Part model, mm, in its own coordinate system. A direction names the side the tool comes from. Round coordinates to 2 decimals unless told otherwise and drop trailing zeros. Order: outer loops, then holes, each group sorted by start corner. A loop starts at its lowest first (then second) coordinate and runs counter-clockwise, first axis right, second up. Notation, with made-up numbers: (88.5, 69) - (124.5, 69) arc R29 ccw to (124.5, 97) - close; hole circle Ø3 at (75.5, 25). An arc over 180 degrees is marked (long way). Return JSON: item names as keys, results as strings. Group by question number.
Item 1: Drop flat-ended pins along their axis: pin 1 (2.5 mm diameter, centred on x = 0, y = 14, fed in from +Z); pin 2 (10 mm diameter, centred on y = -10, z = -13.5, fed in from +X); pin 3 (2 mm diameter, centred on x = -11, z = 2.5, fed in from -Y); pin 4 (4 mm diameter, centred on x = -4, z = -44, fed in from -Y). Give the stop position or say it passes through.
Item 2: Saw through at A-A on x = 0. List the corners of the cut face in (y, z).
Item 3: Probe probe 1 along Z at (x, y) = (-9.5, -1.5); probe 2 along Y at (x, z) = (-16, -24.5); probe 3 along X at (y, z) = (15, -8.5) (3 decimals). List the from-to ranges inside material, lowest first.
Item 4: Saw through at B-B on z = -16. List the corners of the cut face in (x, y).
Item 5: Two-plate mould, pull along Y, no slides. Class faces 4 (the face through (-0.29, -2.23, 13.11)), 5 (the face through (-13.23, -5.986, -1.972)), 6 (the face through (0, -8, -47.5)), 7 (the face through (0, 1.5, 15)): released by +Y, released by -Y, zero draft, split by the parting line, or undercut.
Item 6: Tool access for faces 1 (the face through (-6.963, -2.193, -49.817)), 2 (the face through (0, 0, 23)), 3 (the face through (8, 0, 0)): list every direction of +Z, -Z, +X, -X, +Y, -Y with a clear straight run to the whole face (end or side of a thin tool).
Item 7: Saw through at C-C on z = 18.5. List the corners of the cut face in (x, y).
Autodesk Inventor part; units mm, degrees
ref_plane "YZ Plane" through (0, 0, 0) normal (1, 0, 0) x (0, 1, 0)
ref_plane "XZ Plane" through (0, 0, 0) normal (0, 1, 0) x (-1, 0, 0)
ref_plane "XY Plane" through (0, 0, 0) normal (0, 0, 1) x (1, 0, 0)
sketch "Esquisse1" plane through (0, 0, 0) normal (0, 0, 1) x (1, 0, 0)
  circle A0 centre (0, 0) radius 19.2
  dimension "d0" = 38.4
extrude "Extrusion1" add sketch "Esquisse1" against normal blind 47.5
sketch "Esquisse2" plane through (0, 0, 0) normal (0, 0, 1) x (1, 0, 0)
  circle A0 centre (0, 0) radius 19.2
  circle A1 centre (0, 0) radius 7.5
  dimension "d3" = 15
extrude "Extrusion2" add sketch "Esquisse2" along normal blind 3.5 contours A1
sketch "Esquisse3" plane through (0, 0, 3.5) normal (0, 0, 1) x (1, 0, 0)
  circle A0 centre (0, 0) radius 7.5
  circle A1 centre (0, 0) radius 2.25
  dimension "d6" = 4.5
extrude "Extrusion3" add sketch "Esquisse3" along normal blind 19.5 contours A1
sketch "Esquisse4" plane through (0, 0, -47.5) normal (0, 0, -1) x (-1, 0, 0)
  circle A0 centre (0, 0) radius 19.2
  circle A1 centre (0, 0) radius 7.3
  dimension "d9" = 14.6
extrude "Extrusion4" add sketch "Esquisse4" along normal blind 5.7 contours A1
fillet "Congé1" radius 1 1 edges at (7.3, 0, -53.2)
fillet "Congé2" radius 1 1 edges at (-19.2, 0, 0)
sketch "Esquisse6" plane through (0, 0, 23) normal (0, 0, 1) x (1, 0, 0)
  circle A0 centre (0, 0) radius 2.25
  line L0 (-3, 3.5) -> (3, 3.5)
  line L1 (3, 3.5) -> (3, 1.5)
  line L2 (3, 1.5) -> (-3, 1.5)
  line L3 (-3, 1.5) -> (-3, 3.5)
  dimension "d14" = 1.5
  dimension "d15" = 2
  dimension "d16" = 6
  dimension "d17" = 3
extrude "Extrusion5" cut sketch "Esquisse6" against normal blind 17 contours L2 A0 | A0 L2 L3 L0 L1 picked at (-0.424, 1.6187)
sketch "Esquisse7" plane through (0, 0, 0) normal (0, 0, 1) x (1, 0, 0)
  circle A0 centre (0, 0) radius 7.5
  circle A1 centre (0, 14) radius 1.5
  dimension "d20" = 3
  dimension "d21" = 14
extrude "Extrusion6" cut sketch "Esquisse7" against normal blind 4 contours A1
thread "Filetage1"
pattern_circular "Réseau circulaire1" count 3 over 360 about axis through (0, 0, 0) along (0, 0, -1) of "Extrusion6"
thread "Filetage2"
thread "Filetage3"
equation "\"d17\" = 0.5 * d16"
properties part number "Nidec_DMN37"
Filled in:
{
 "1": {"pin 1": "stops at z = -4", "pin 2": "stops at x = 18.54", "pin 3": "passes through", "pin 4": "stops at y = -19.1"},
 "2": {"outline": "(-19.2, -47.5) - (-7.3, -47.5) - (-7.3, -52.2) arc R1 ccw to (-6.3, -53.2) - (6.3, -53.2) arc R1 ccw to (7.3, -52.2) - (7.3, -47.5) - (19.2, -47.5) - (19.2, -1) arc R1 ccw to (18.2, 0) - (15.5, 0) - (15.5, -4) - (12.5, -4) - (12.5, 0) - (7.5, 0) - (7.5, 3.5) - (2.25, 3.5) - (2.25, 6) - (1.5, 6) - (1.5, 23) - (-2.25, 23) - (-2.25, 3.5) - (-7.5, 3.5) - (-7.5, 0) - (-18.2, 0) arc R1 ccw to (-19.2, -1) - close"},
 "3": {"probe 1": "z = -47.5 to 0", "probe 2": "y = -10.61 to 10.61", "probe 3": "x = -11.985 to 11.985"},
 "4": {"outline": "circle Ø38.4 at (0, 0)"},
 "5": {"face 4": "split by the parting line", "face 5": "undercut", "face 6": "zero draft", "face 7": "released by +Y"},
 "6": {"face 1": "-Z", "face 2": "+Z, +X, -X, +Y, -Y", "face 3": "+Z"},
 "7": {"outline": "(-1.68, 1.5) arc R2.25 ccw (long way) to (1.68, 1.5) - close"}
}
